Here's the drawing with two shaded views (mm, measured from the low corner). I have some questions. A direction names the side the tool comes from. Coordinates: 2 decimals unless noted, no trailing zeros. Write each loop counter-clockwise with the first axis right and the second up, starting at its lowest first coordinate (ties: lowest second). Pieces come first, ordered by that corner, then holes. Notation, with made-up numbers: M 54.25,28 L 83.25,28 A7 ccw 83.25,35 Z; hole C 65.25,68.5 d3. An arc over 180 degrees is marked long. Answer as CSV lines item,"result". Start each with the question number.
Item 1: Suppose I cut it at B-B, the plane x = 3. Write out the boundary of the cut face in (y, z).
Item 2: Suppose I cut it at D-D, the plane x = 25. Write out the boundary of the cut face in (y, z), and give its area (3 significant figures).
Item 3: Suppose I cut it at C-C, the plane z = 24. Write out the boundary of the cut face in (x, y).
Item 4: If I drill on line 1 along X through (y, z) = (0.75, 24); line 2 along Y through (x, z) = (3, 1.1); line 3 along Z through (x, y) = (26.5, 27.5), over which ranges is the centre line in solid material (lowest first)? Write a range as [from, to].
Item 5: I'm going to push flat-ended pins straight in: P1, Ø6, axis at y = 14.5, z = 4.5, coming from the +X side; P2, Ø1.6, axis at y = 39, z = 0.5, coming from the -X side; P3, Ø1.6, axis at x = 41.5, y = 0.5, coming from the -Z side. Where does each tip first touch, or does it pass through?
Item 6: Suppose I cut it at A-A, the plane y = 41.5. Write out the boundary of the cut face in (x, z).
Item 7: On a 3-axis mill with a long thin cutter (end or side, diameter ignored), from which of +Z, -Z, +X, -X, +Y, -Y can I reach the whole of each face in a straight line? I mean the marked faces 1 and 2. Say none if no direction works.
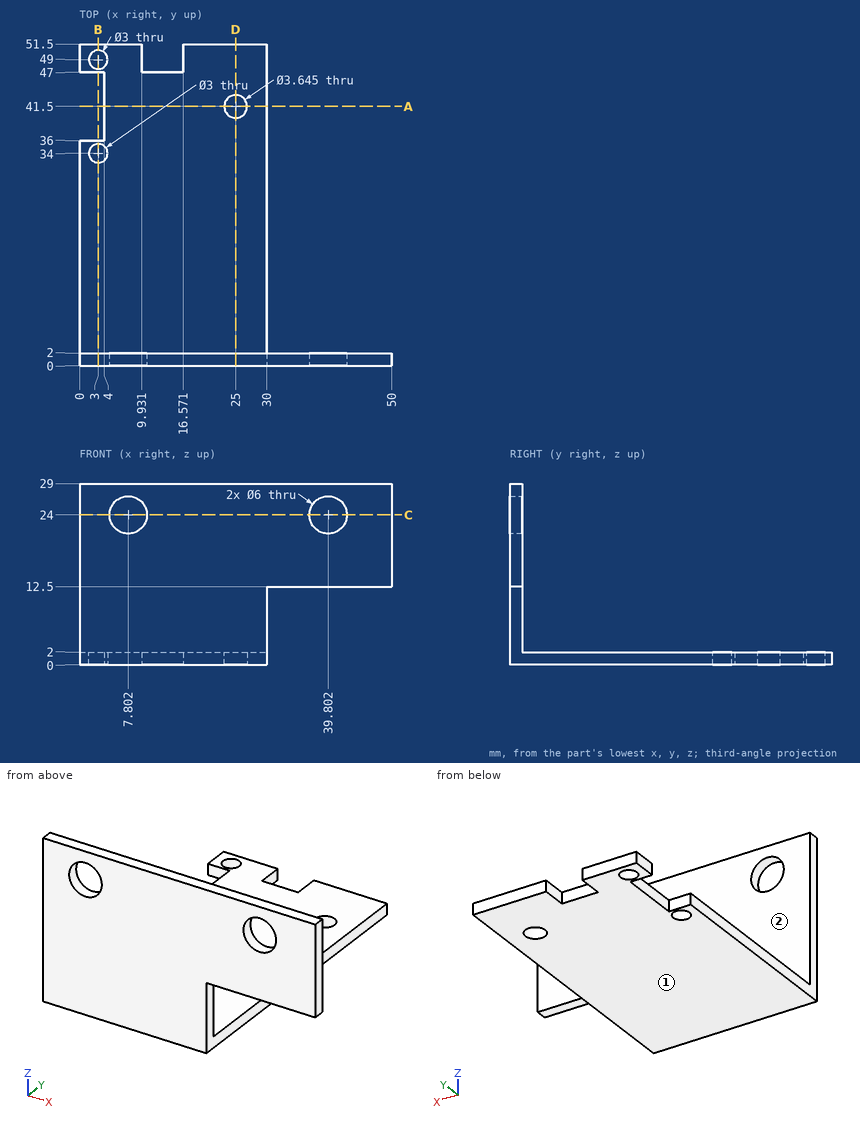
Ans:
1,outline,"M 0,0 L 32.5,0 L 32.5,2 L 2,2 L 2,29 L 0,29 Z; M 35.5,0 L 36,0 L 36,2 L 35.5,2 Z; M 47,0 L 47.5,0 L 47.5,2 L 47,2 Z; M 50.5,0 L 51.5,0 L 51.5,2 L 50.5,2 Z"
2,outline,"M 0,0 L 39.68,0 L 39.68,2 L 2,2 L 2,29 L 0,29 Z; M 43.32,0 L 51.5,0 L 51.5,2 L 43.32,2 Z"
2,area,"150 mm^2"
3,outline,"M 0,0 L 4.8,0 L 4.8,2 L 0,2 Z; M 10.8,0 L 36.8,0 L 36.8,2 L 10.8,2 Z; M 42.8,0 L 50,0 L 50,2 L 42.8,2 Z"
4,line 1,"x = [0, 4.8], [10.8, 36.8], [42.8, 50]"
4,line 2,"y = [0, 32.5], [35.5, 36], [47, 47.5], [50.5, 51.5]"
4,line 3,"z = [0, 2]"
5,P1,"stops at x = 30"
5,P2,"stops at x = 4"
5,P3,"stops at z = 12.5"
6,outline,"M 4,0 L 23.18,0 L 23.18,2 L 4,2 Z; M 26.82,0 L 30,0 L 30,2 L 26.82,2 Z"
7,face 1,"-Z, +X, -X, +Y, -Y"
7,face 2,"+Z, +X, -X, +Y"
